```python
from build123d import *

# Parameters (mm, degrees)
F0_W        = 15.24
F0_H        = 12.7
F1_DEPTH    = 5.08
F2_T1_DEPTH = 15.24
F2_T3_DEPTH = 19.4141495789


# Not quite as in the source:
# - a fillet or chamfer that OpenCascade refuses, or shapes differently, is made with other operations: its cross-section is extruded or revolved along the edge and cut away or added
# - a feature names something its author has since deleted; it is built from what else it names


with BuildPart() as f1:
    # F0 (on Top) → F1 (new body)
    with BuildSketch(Plane.XY):
        Polygon((-43.6893899012, 21.153706044), (-37.9743899012, 21.153706044), (-34.7993899012, 21.153706044), (-31.6243899012, 21.153706044), (-25.9093899012, 21.153706044), (-25.9093899012, 38.933706044), (-43.6893899012, 38.933706044), align=None)
        with Locations((-34.6747071493, 29.6888263732)):
            Rectangle(F0_W, F0_H, mode=Mode.SUBTRACT)
        Polygon((-34.7993899012, 21.153706044), (-37.9743899012, 21.153706044), (-37.9743899012, -42.346293956), (-31.6243899012, -42.346293956), (-31.6243899012, 21.153706044), align=None)
    extrude(amount=F1_DEPTH)

    # F2: chamfer of 2.54 on 4 edges, made by hand

    # F2_s2 → F2_t1 (cut)
    with BuildSketch(Plane.YZ.offset(-42.2947071493)):
        Polygon((36.0388263732, 2.54), (38.5788263732, 5.08), (36.0388263732, 5.08), align=None)
        Polygon((23.3388263732, 2.54), (20.7988263732, 5.08), (23.3388263732, 5.08), align=None)
    extrude(amount=F2_T1_DEPTH, mode=Mode.SUBTRACT)

    # F2_s4 → F2_t3 (cut)
    with BuildSketch(Plane.YZ.offset(-44.5064646906)):
        Polygon((-42.346293956, 2.54), (-39.806293956, 5.08), (-42.346293956, 5.08), align=None)
        Polygon((-42.346293956, 2.54), (-39.806293956, 0), (-42.346293956, 0), align=None)
    extrude(amount=F2_T3_DEPTH, mode=Mode.SUBTRACT)


solid = f1.part
```
Design review of the part built by this model. Coordinates are the model's own, in mm. A direction names the side the tool comes from. Coordinates: 2 decimals unless noted, no trailing zeros. Loops run counter-clockwise (first coordinate to the right, second up) from the corner with the lowest first, then second, coordinate; pieces in that order, holes last. Notation, with made-up numbers: (32.25, -37) - (37.25, -37) arc R17 cw to (37.25, -33) - close; hole circle Ø3 at (22.25, 14). An arc over 180 degrees is marked (long way). Use CSV: the item, a comma, the result in double quotes. Start each with the question number.
1) Consider section C-C on y = 17. Write out the cut boundary in (x, z).
2) The part is to be moulded in two halves that separate along Y. For faces 4 (the flat face through (-35, -9, 5.08)), 5 (the flat face through (-41, 21.154, 3)), 6 (the flat face through (-27.055, 30, 3)), say which applies: +Y half, -Y half, draft (parallel to the pull), parting line (faces both ways), or undercut.
3) For pin 1 Ø2.5 at (x, z) = (-28.5, 2) entering from -Y, flat-tipped, find the tip position at first contact; note if it passes through.
4) Wall thickness on L1, parallel to Y at x = -27.75, z = 0.3; L2, parallel to X at y = 31, z = 2.3; L3, parallel to X at y = -9.5, z = 2.2: over which ranges is each line inside the solid? List them lowest first. Write a range as from..to.
5) Consider section A-A on x = -37. Write out the cut boundary in (y, z).
6) Tool access review of faces 1 (the flat face through (-34.78, 22.09, 3.79)), 2 (the flat face through (-31.624, -11, 3)), 3 (the flat face through (-35, 23.339, 1)): name each direction out of +Z, -Z, +X, -X, +Y, -Y from which nothing blocks a thin tool from reaching the whole face with its end or side.
7) Consider section B-B on z = 0.9. Write out the cut boundary in (x, y).
Geometry says:
1,outline,"(-37.97, 0) - (-31.62, 0) - (-31.62, 5.08) - (-37.97, 5.08) - close"
2,face 4,"draft"
2,face 5,"-Y half"
2,face 6,"undercut"
3,pin 1,"y = 21.15"
4,L1,"21.15..23.34, 36.04..38.93"
4,L2,"-43.69..-42.29, -27.05..-25.91"
4,L3,"-37.97..-31.62"
5,outline,"(-42.35, 2.54) - (-39.81, 0) - (23.34, 0) - (23.34, 2.54) - (20.8, 5.08) - (-39.81, 5.08) - close; (36.04, 0) - (38.93, 0) - (38.93, 5.08) - (38.58, 5.08) - (36.04, 2.54) - close"
6,face 1,"+Z"
6,face 2,"+Z, -Z, +X, -Y"
6,face 3,"+Z, -Z"
7,outline,"(-43.69, 21.15) - (-37.97, 21.15) - (-37.97, -40.71) - (-31.62, -40.71) - (-31.62, 21.15) - (-25.91, 21.15) - (-25.91, 38.93) - (-43.69, 38.93) - close; hole (-42.29, 23.34) - (-27.05, 23.34) - (-27.05, 36.04) - (-42.29, 36.04) - close"
